Source: CAD feature listing. Evaluate the final solid. Frame: model axes, mm. Face numbers are marked on the shaded views. Round coordinates to 2 decimals unless told otherwise and drop trailing zeros. One line per item, written item: value. Start each with the question number.
1) Mould query, pull axis X, two halves, no side actions, for the marked faces 1 and 2. Classes: pulls with the +X half, pulls with the -X half, needs draft (parallel to the pull), parting line crosses it, or undercut.
2) Section A-A (z = 8.5). State how many separate pieces and enclosed holes the cut face has, and give its area (3 significant figures).
3) Pin query (flat end, axial travel): P1, Ø4, axis at x = 90.18, y = -37.49, coming from the -Z side; P2, Ø1.5, axis at x = 23, z = 2, coming from the +Y side; P3, Ø3.5, axis at x = 35.24, y = 12.83, coming from the +Z side; P4, Ø3, axis at y = -36.5, z = 1.5, coming from the -X side. Return the tip coordinate at first contact, or that it passes through.
4) Ray query, L1, parallel to X at y = -20.5, z = 7.25; L2, parallel to X at y = -30, z = 7.5; L3, parallel to Y at x = 4, z = 7.5. Return the intervals inside material, ascending.
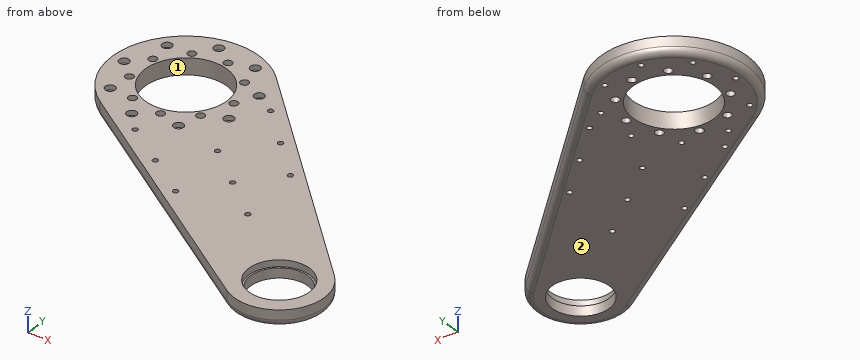
```python
from build123d import *

# Parameters (mm, degrees)
SKETCH1_R           = 17.5
SKETCH1_R_2         = 1.6
BOSS_EXTRUDE1_DEPTH = 10
SKETCH2_R           = 25
SKETCH2_R_2         = 2.5
SKETCH2_R_3         = 1.6
CUT_EXTRUDE1_DEPTH  = 224.991888552
SKETCH3_R           = 18.5625
CUT_EXTRUDE2_DEPTH  = 4
SKETCH4_R           = 3
CUT_EXTRUDE3_DEPTH  = 3
FILLET1_R           = 4


with BuildPart() as part:
    # Sketch1 → Boss-Extrude1 (new body)
    with BuildSketch(Plane.XY):
        with BuildLine():
            Line((-25.534872354, -37.053613776), (126.113577761, -141.559582877))
            ThreePointArc((126.113577761, -141.559582877), (162.784444163, -136.592367058), (161.308367688, -99.616065541))
            Line((161.308367688, -99.616065541), (32.056602073, 31.581232775))
            ThreePointArc((32.056602073, 31.581232775), (-34.47199994, 28.925442436), (-25.534872354, -37.053613776))
        make_face()
        with Locations((141.718221977, -118.915707792)):
            Circle(SKETCH1_R, mode=Mode.SUBTRACT)
        with Locations((70.859110989, -59.457853896)):
            Circle(SKETCH1_R_2, mode=Mode.SUBTRACT)
        with Locations((93.840444282, -78.741482187)):
            Circle(SKETCH1_R_2, mode=Mode.SUBTRACT)
        with Locations((47.877777695, -40.174225605)):
            Circle(SKETCH1_R_2, mode=Mode.SUBTRACT)
        with Locations((47.767990244, 4.946625931)):
            Circle(SKETCH1_R_2, mode=Mode.SUBTRACT)
        with Locations((3.423348889, -47.901259716)):
            Circle(SKETCH1_R_2, mode=Mode.SUBTRACT)
        with Locations((68.973861607, -16.273907044)):
            Circle(SKETCH1_R_2, mode=Mode.SUBTRACT)
        with Locations((90.17973297, -37.494440018)):
            Circle(SKETCH1_R_2, mode=Mode.SUBTRACT)
        with Locations((28.003855203, -65.100059364)):
            Circle(SKETCH1_R_2, mode=Mode.SUBTRACT)
        with Locations((52.584361518, -82.298859012)):
            Circle(SKETCH1_R_2, mode=Mode.SUBTRACT)
    extrude(amount=BOSS_EXTRUDE1_DEPTH)

    # Sketch2 → Cut-Extrude1 (cut, through all)
    with BuildSketch(Plane.XY.offset(10)):
        Circle(SKETCH2_R)
        with Locations((29, 0)):
            Circle(SKETCH2_R_2)
        with Locations((-37.5, 0)):
            Circle(SKETCH2_R_3)
        with Locations((-28.726666617, 24.104535363)):
            Circle(SKETCH2_R_3)
        with Locations((-6.511806663, 36.930290738)):
            Circle(SKETCH2_R_3)
        with Locations((18.75, 32.475952642)):
            Circle(SKETCH2_R_3)
        with Locations((35.238473279, 12.825755375)):
            Circle(SKETCH2_R_3)
        with Locations((35.238473279, -12.825755375)):
            Circle(SKETCH2_R_3)
        with Locations((18.75, -32.475952642)):
            Circle(SKETCH2_R_3)
        with Locations((-6.511806663, -36.930290738)):
            Circle(SKETCH2_R_3)
        with Locations((-28.726666617, -24.104535363)):
            Circle(SKETCH2_R_3)
        with Locations((22.21528885, -18.640840681)):
            Circle(SKETCH2_R_2)
        with Locations((5.035797152, -28.559424837)):
            Circle(SKETCH2_R_2)
        with Locations((-14.5, -25.11473671)):
            Circle(SKETCH2_R_2)
        with Locations((-27.251086003, -9.918584156)):
            Circle(SKETCH2_R_2)
        with Locations((-27.251086003, 9.918584156)):
            Circle(SKETCH2_R_2)
        with Locations((-14.5, 25.11473671)):
            Circle(SKETCH2_R_2)
        with Locations((5.035797152, 28.559424837)):
            Circle(SKETCH2_R_2)
        with Locations((22.21528885, 18.640840681)):
            Circle(SKETCH2_R_2)
    extrude(amount=-CUT_EXTRUDE1_DEPTH, mode=Mode.SUBTRACT)

    # Sketch3 → Cut-Extrude2 (cut)
    with BuildSketch(Plane.XY.offset(10)):
        with Locations((141.718221977, -118.915707792)):
            Circle(SKETCH3_R)
    extrude(amount=-CUT_EXTRUDE2_DEPTH, mode=Mode.SUBTRACT)

    # Sketch4 → Cut-Extrude3 (cut)
    with BuildSketch(Plane.XY.offset(10)):
        with Locations((-28.726666617, 24.104535363)):
            Circle(SKETCH4_R)
        with Locations((-6.511806663, 36.930290738)):
            Circle(SKETCH4_R)
        with Locations((18.75, 32.475952642)):
            Circle(SKETCH4_R)
        with Locations((35.238473279, 12.825755375)):
            Circle(SKETCH4_R)
        with Locations((35.238473279, -12.825755375)):
            Circle(SKETCH4_R)
        with Locations((18.75, -32.475952642)):
            Circle(SKETCH4_R)
        with Locations((-6.511806663, -36.930290738)):
            Circle(SKETCH4_R)
        with Locations((-28.726666617, -24.104535363)):
            Circle(SKETCH4_R)
        with Locations((-37.5, 0)):
            Circle(SKETCH4_R)
    extrude(amount=-CUT_EXTRUDE3_DEPTH, mode=Mode.SUBTRACT)

    # Fillet1
    fillet1_edges = [part.edges().sort_by_distance(p)[0] for p in [
        (96.68248488, -34.017416383, 0),
        (162.784444163, -136.592367058, 0),
        (50.289352703, -89.306598327, 0),
        (-34.47199994, 28.925442436, 0),
    ]]
    fillet(fillet1_edges, radius=FILLET1_R)


solid = part.part
```
Findings:
1. face 1: undercut
1. face 2: needs draft
2. separate pieces: 1
2. enclosed holes: 29
2. area: 14,300 mm2
3. P1: z = 0
3. P2: y = 38.67
3. P3: z = 7
3. P4: x = -27.38
4. L1: -40.06 to -14.31, 14.31 to 20.54, 23.89 to 83.37
4. L2: -33.54 to 2.99, 7.08 to 17.06, 20.44 to 92.72
4. L3: -57.41 to -49.39, -46.41 to -30.83, -26.28 to -24.68, 24.68 to 26.28, 30.83 to 44.82
